from build123d import *

# Parameters (mm, degrees)
CROQUIS1_W              = 290
CROQUIS1_H              = 164
SALIENTE_EXTRUIR1_DEPTH = 172
REDONDEO1_R             = 10
VACIADO1_START          = -135
VACIADO1_OUTLINE_W      = 154
VACIADO1_OUTLINE_H      = 152
VACIADO1_DEPTH          = 270
REDONDEO2_R             = 10


# Read off the part's stored shape, not the designer's step: Vaciado1
with BuildPart() as part:
    # Croquis1 → Saliente-Extruir1 (new body)
    with BuildSketch(Plane.XY):
        Rectangle(CROQUIS1_W, CROQUIS1_H)
    extrude(amount=SALIENTE_EXTRUIR1_DEPTH)

    # Redondeo1
    redondeo1_edges = [part.edges().sort_by_distance(p)[0] for p in [
        (-145, 0, 172),
        (145, 0, 172),
        (-145, 0, 0),
        (145, 0, 0),
    ]]
    fillet(redondeo1_edges, radius=REDONDEO1_R)

    # Vaciado1 outline → Vaciado1 (cut)
    with BuildSketch(Plane.YZ.offset(VACIADO1_START)):
        with Locations((5, 86)):
            Rectangle(VACIADO1_OUTLINE_W, VACIADO1_OUTLINE_H)
    extrude(amount=VACIADO1_DEPTH, mode=Mode.SUBTRACT)

    # Redondeo2
    redondeo2_edges = [part.edges().sort_by_distance(p)[0] for p in [
        (135, 5, 162),
        (-135, 5, 162),
        (-135, 5, 10),
        (135, 5, 10),
    ]]
    fillet(redondeo2_edges, radius=REDONDEO2_R)


solid = part.part
Check sheet for the modelled part. Datum: model origin and axes. Units: mm. A direction names the side the tool comes from. Give positions to 0.01 mm unless a question says otherwise; leave off trailing zeros. Loops run counter-clockwise (first coordinate to the right, second up) from the corner with the lowest first, then second, coordinate; pieces in that order, holes last. Notation, with made-up numbers: M 57.25,23.5 L 77.25,23.5 A16 ccw 77.25,27.5 Z; hole C 52,-27 d10. An arc over 180 degrees is marked long. Use a Markdown table: item, result. Add a question column.
Q1. Sectioned sample at B-B, the plane x = -111. Record the cut outline in (y, z), then the cut area to 3 significant figures.
Q2. Tool access check on faces 4 (the flat face through (-2, 4, 10)), 5 (the flat face through (-2, 1, 0)). Record the directions out of +Z, -Z, +X, -X, +Y, -Y that give a thin tool (end or side, any length) a straight path to the whole face; none if there is none.
Q3. Mould release check, pull along X, two halves, no side actions. Record for faces 1 (the flat face through (-2, -82, 85)), 2 (the cylindrical face through (142.15, 1.15, 168.99)), 3 (the flat face through (-135, 4, 87)): pulls with the +X half, pulls with the -X half, needs draft (parallel to the pull), parting line crosses it, or undercut.
Q4. Sectioned sample at A-A, the plane y = -67. Record the cut outline in (x, z), then the cut area to 3 significant figures.
Q5. Go/stop test with a flat-tipped pin: pin 1 (4 mm diameter, centred on x = -75.5, z = 149, fed in from +Y). Record where the tip stops, or that it passes through.
Q6. Scan lines: line 1 along Z through (x, y) = (-14, 1.5); line 2 along X through (y, z) = (8, 53.5); line 3 along Y through (x, z) = (88.5, 67). Record each from-to range of solid material in increasing order. Write a range as [from, to].
Q7. Sectioned sample at C-C, the plane z = 90.5. Record the cut outline in (x, y), then the cut area to 3 significant figures.
Verdict:
| question | item | result |
|---|---|---|
| 1 | outline | M -82,0 L 82,0 L 82,10 L -72,10 L -72,162 L 82,162 L 82,172 L -82,172 Z |
| 1 | area | 4,800 mm^2 |
| 2 | face 4 | +Y |
| 2 | face 5 | -Z, +X, -X, +Y, -Y |
| 3 | face 1 | needs draft |
| 3 | face 2 | pulls with the +X half |
| 3 | face 3 | undercut |
| 4 | outline | M -145,10 A10 ccw -135,0 L 135,0 A10 ccw 145,10 L 145,162 A10 ccw 135,172 L -135,172 A10 ccw -145,162 Z; hole M -135,20 A10 ccw -125,10 L 125,10 A10 ccw 135,20 L 135,152 A10 ccw 125,162 L -125,162 A10 ccw -135,152 Z |
| 4 | area | 8,840 mm^2 |
| 5 | pin 1 | y = -72 |
| 6 | line 1 | [0, 10], [162, 172] |
| 6 | line 2 | [-145, -135], [135, 145] |
| 6 | line 3 | [-82, -72] |
| 7 | outline | M -145,-82 L 145,-82 L 145,82 L 135,82 L 135,-72 L -135,-72 L -135,82 L -145,82 Z |
| 7 | area | 5,980 mm^2 |
